Check sheet for the modelled part. Datum: model origin and axes. Units: mm. A direction names the side the tool comes from. Round coordinates to 2 decimals unless told otherwise and drop trailing zeros. Order: outer loops, then holes, each group sorted by start corner. A loop starts at its lowest first (then second) coordinate and runs counter-clockwise, first axis right, second up. Notation, with made-up numbers: (87.25, 74.5) -> (94.25, 74.5) arc R33 ccw to (94.25, 110.5) -> close; hole circle Ø7 at (43.25, -23.5). An arc over 180 degrees is marked (long way). Use CSV: the item, a comma, the result in double quotes.
```python
from build123d import *

# Parameters (mm, degrees)
BOSS_EXTRUDE1_DEPTH = 3
SKETCH2_R           = 1.7
CUT_EXTRUDE1_DEPTH  = 3
BOSS_EXTRUDE2_DEPTH = 2
SKETCH6_R           = 1.8
CUT_EXTRUDE2_DEPTH  = 3
SKETCH8_W           = 10.85
SKETCH8_H           = 1.4
CUT_EXTRUDE4_DEPTH  = 1.3
FILLET2_R           = 0.5


with BuildPart() as part:
    # Sketch1 → Boss-Extrude1 (new body)
    with BuildSketch(Plane.XY):
        with BuildLine():
            Line((-16.06, -32.453666973), (16.06, -32.453666973))
            ThreePointArc((16.06, -32.453666973), (0, 36.21), (-16.06, -32.453666973))
        make_face()
    extrude(amount=BOSS_EXTRUDE1_DEPTH)

    # Sketch2 → Cut-Extrude1 (cut)
    with BuildSketch(Plane.XY.offset(3)):
        with Locations((-20.955, 21.12)):
            Circle(SKETCH2_R)
        with Locations((20.955, 21.12)):
            Circle(SKETCH2_R)
        with Locations((-20.955, -21.12)):
            Circle(SKETCH2_R)
        with Locations((20.955, -21.12)):
            Circle(SKETCH2_R)
    extrude(amount=-CUT_EXTRUDE1_DEPTH, mode=Mode.SUBTRACT)

    # Sketch4 → Boss-Extrude2 (add)
    with BuildSketch(Plane.XY.offset(3)):
        with BuildLine():
            Line((-17.534144761, 28.989794195), (-16.499071281, 27.278472224))
            ThreePointArc((-16.499071281, 27.278472224), (0, 31.88), (16.499071281, 27.278472224))
            Line((16.499071281, 27.278472224), (17.534144761, 28.989794195))
            ThreePointArc((17.534144761, 28.989794195), (0, 33.88), (-17.534144761, 28.989794195))
        make_face()
        with BuildLine():
            Line((-28.851381969, 17.760972903), (-27.148230731, 16.712509332))
            ThreePointArc((-27.148230731, 16.712509332), (-31.88, 0), (-27.148230731, -16.712509332))
            Line((-27.148230731, -16.712509332), (-28.851381969, -17.760972903))
            ThreePointArc((-28.851381969, -17.760972903), (-33.88, 0), (-28.851381969, 17.760972903))
        make_face()
        with BuildLine():
            Line((28.851381969, 17.760972903), (27.148230731, 16.712509332))
            ThreePointArc((27.148230731, 16.712509332), (31.88, 0), (27.148230731, -16.712509332))
            Line((27.148230731, -16.712509332), (28.851381969, -17.760972903))
            ThreePointArc((28.851381969, -17.760972903), (33.88, 0), (28.851381969, 17.760972903))
        make_face()
    extrude(amount=BOSS_EXTRUDE2_DEPTH)

    # Sketch6 → Cut-Extrude2 (cut)
    with BuildSketch(Plane(origin=(0, 0, 0), x_dir=(-1, 0, 0), z_dir=(0, 0, -1))):
        with Locations((9.56, -22.453666973)):
            Circle(SKETCH6_R)
        with Locations((9.56, -26.523666973)):
            Circle(SKETCH6_R)
    extrude(amount=-CUT_EXTRUDE2_DEPTH, mode=Mode.SUBTRACT)

    # Sketch8 → Cut-Extrude4 (cut)
    with BuildSketch(Plane.XY.offset(3)):
        with Locations((8.635, -30.753666973)):
            Rectangle(SKETCH8_W, SKETCH8_H)
    extrude(amount=-CUT_EXTRUDE4_DEPTH, mode=Mode.SUBTRACT)

    # Fillet2
    fillet2_edges = [part.edges().sort_by_distance(p)[0] for p in [
        (-7.76, -22.453666973, 3),
    ]]
    fillet(fillet2_edges, radius=FILLET2_R)


solid = part.part
```
Q1. Go/stop test with flat-tipped pins: pin 1 (3 mm diameter, centred on x = 19, z = 3.5, fed in from +Y); pin 2 (10 mm diameter, centred on x = -1, y = 26.5, fed in from +Z); pin 3 (6 mm diameter, centred on x = -9.56, y = -22.45, fed in from -Z); pin 4 (1 mm diameter, centred on y = -31, z = 2, fed in from +X). Record where each tip stops, or that it passes through.
Result sheet:
pin 1,"stops at y = 31.65"
pin 2,"stops at z = 3"
pin 3,"stops at z = 0"
pin 4,"stops at x = 19.52"
Q2. Access from +Z, -Z, +X, -X, +Y, -Y to the whole of each face (thin tool, end or side, straight path). Record for faces 5 (the face through (-31.88, 0.25, 3.99)), 6 (the face through (-17.024, 28.146, 3.986)), 7 (the face through (-32.2, 0.1, 5)), 8 (the face through (27.99, -17.23, 3.99)), 9 (the face through (28.012, 17.244, 3.986)).
Result sheet:
face 5,"+Z"
face 6,"+Z, -X, -Y"
face 7,"+Z, +X, -X, +Y, -Y"
face 8,"+Z, -Y"
face 9,"+Z, +Y"
Q3. Scan lines: L1, parallel to Y at x = -21.5, z = 0.3; L2, parallel to Z at x = -2, y = 8; L3, parallel to X at y = 8, z = 4.55. Record each from-to range of solid material in increasing order.
Result sheet:
L1,"y = -29.14 to -22.73, -19.51 to 19.51, 22.73 to 29.14"
L2,"z = 0 to 3"
L3,"x = -32.92 to -30.86, 30.86 to 32.92"
Q4. Sectioned sample at D-D, the plane x = 11. Enter the section's corners in (y, z).
Result sheet:
outline,"(-32.45, 0) -> (34.5, 0) -> (34.5, 3) -> (32.04, 3) -> (32.04, 5) -> (29.92, 5) -> (29.92, 3) -> (-30.05, 3) -> (-30.05, 1.7) -> (-31.45, 1.7) -> (-31.45, 3) -> (-32.45, 3) -> close"
Q5. Sectioned sample at C-C, the plane y = -1. Enter the section's corners in (x, z).
Result sheet:
outline,"(-36.2, 0) -> (36.2, 0) -> (36.2, 3) -> (33.87, 3) -> (33.87, 5) -> (31.86, 5) -> (31.86, 3) -> (-31.86, 3) -> (-31.86, 5) -> (-33.87, 5) -> (-33.87, 3) -> (-36.2, 3) -> close"
Q6. Sectioned sample at B-B, the plane x = -21.5. Enter the section's corners in (y, z), then the cut area to 3 significant figures.
Result sheet:
outline,"(-29.14, 0) -> (-22.73, 0) -> (-22.73, 3) -> (-29.14, 3) -> close; (-19.51, 0) -> (19.51, 0) -> (19.51, 3) -> (-19.51, 3) -> close; (22.73, 0) -> (29.14, 0) -> (29.14, 3) -> (22.73, 3) -> close"
area,"155 mm^2"
Q7. Mould release check, pull along Y, two halves, no side actions. Record for faces 1 (the face through (-27.99, -17.23, 3.99)), 2 (the face through (-19.385, 20.469, 1.521)), 3 (the face through (-1, 2, 0)), 4 (the face through (33.88, -0.26, 3.99)): pulls with the +Y half, pulls with the -Y half, needs draft (parallel to the pull), parting line crosses it, or undercut.
Result sheet:
face 1,"pulls with the -Y half"
face 2,"undercut"
face 3,"needs draft"
face 4,"parting line crosses it"
Q8. Sectioned sample at A-A, the plane z = 3.95. Enter the section's corners in (x, y).
Result sheet:
outline,"(-28.85, -17.76) -> (-27.15, -16.71) arc R31.88 cw to (-27.15, 16.71) -> (-28.85, 17.76) arc R33.88 ccw to start; (-17.53, 28.99) -> (-16.5, 27.28) arc R31.88 cw to (16.5, 27.28) -> (17.53, 28.99) arc R33.88 ccw to start; (27.15, -16.71) -> (28.85, -17.76) arc R33.88 ccw to (28.85, 17.76) -> (27.15, 16.71) arc R31.88 cw to start"
